from build123d import *

# Parameters (mm, degrees)
F0_W     = 31.419306
F0_H     = 12.7
F1_DEPTH = 66.83598


with BuildPart() as f1:
    # F0 (on Top) → F1 (new body)
    with BuildSketch(Plane.XY):
        Polygon((-99.093348, 73.004946), (-111.793348, 73.004946), (-111.793348, -77.210762), (-99.093348, -77.210762), (-99.093348, -5.429364), (-99.093348, 7.270636), align=None)
        with Locations((-83.383695, 0.920636)):
            Rectangle(F0_W, F0_H)
        Polygon((-67.674042, 73.004946), (-67.674042, 7.270636), (-67.674042, -5.429364), (-67.674042, -77.210762), (-54.974042, -77.210762), (-54.974042, 73.004946), align=None)
    extrude(amount=F1_DEPTH)


solid = f1.part
Can you work these out from the model? Positions are in its coordinate system, mm. A direction names the side the tool comes from. Round coordinates to 2 decimals unless told otherwise and drop trailing zeros. Write each loop counter-clockwise with the first axis right and the second up, starting at its lowest first coordinate (ties: lowest second). Pieces come first, ordered by that corner, then holes. Notation, with made-up numbers: (-1, 31) -> (57, 31) arc R11 cw to (57, 45) -> close; hole circle Ø6 at (53, 31). An arc over 180 degrees is marked (long way). One line per question, with ' | ' between items. Start each with the question number.
1) I'm going to push flat-ended pins straight in: P1, Ø8, axis at x = -69, y = -21, coming from the +Z side; P2, Ø9.5, axis at x = -83.5, z = 44, coming from the -Y side. Where does each tip first touch, or does it pass through?
2) I need wall thicknesses on line 1 (X direction, y = -18, z = 15); line 2 (Y direction, x = -98, z = 12.5). Which ranges of each line are inside material? Lowest first, please. Write a range as [from, to].
3) Suppose I cut it at C-C on x = -89.5. Write out the boundary of the cut face in (y, z).
4) On a 3-axis mill with a long thin cutter (end or side, diameter ignored), from which of +Z, -Z, +X, -X, +Y, -Y can I reach the whole of each face in a straight line? I mean faces 1 (the flat face through (-61, 73.005, 33)), 2 (the flat face through (-67.674, 41, 33)), 3 (the flat face through (-99.093, -42, 33)). Say none if no direction works.
5) Suppose I cut it at A-A on y = -31. Write out the boundary of the cut face in (x, z), then the cut area to 3 significant figures.
6) If we mould it in two halves opening along X, with no side actions, what happens to faces 4 (the flat face through (-84, -1, 0)), 5 (the flat face through (-84, -5.429, 33)), 6 (the flat face through (-54.974, -3, 33))? For each: released by +X, released by -X, zero draft, split by the parting line, or undercut.
7) Suppose I cut it at B-B on z = 61. Write out the boundary of the cut face in (x, y).
Return value:
1) P1: stops at z = 66.84 | P2: stops at y = -5.43
2) line 1: x = [-111.79, -99.09], [-67.67, -54.97] | line 2: y = [-5.43, 7.27]
3) outline: (-5.43, 0) -> (7.27, 0) -> (7.27, 66.84) -> (-5.43, 66.84) -> close
4) face 1: +Z, -Z, +X, -X, +Y | face 2: +Z, -Z, +Y | face 3: +Z, -Z, -Y
5) outline: (-111.79, 0) -> (-99.09, 0) -> (-99.09, 66.84) -> (-111.79, 66.84) -> close; (-67.67, 0) -> (-54.97, 0) -> (-54.97, 66.84) -> (-67.67, 66.84) -> close | area: 1,700 mm2
6) face 4: zero draft | face 5: undercut | face 6: released by +X
7) outline: (-111.79, -77.21) -> (-99.09, -77.21) -> (-99.09, -5.43) -> (-67.67, -5.43) -> (-67.67, -77.21) -> (-54.97, -77.21) -> (-54.97, 73) -> (-67.67, 73) -> (-67.67, 7.27) -> (-99.09, 7.27) -> (-99.09, 73) -> (-111.79, 73) -> close
